Read the model definition and answer for the solid it produces. Units are mm, in the model's axes. Face numbers are marked on the shaded views. A direction names the side the tool comes from. Give positions to 0.01 mm unless a question says otherwise; leave off trailing zeros. Order: outer loops, then holes, each group sorted by start corner. A loop starts at its lowest first (then second) coordinate and runs counter-clockwise, first axis right, second up.
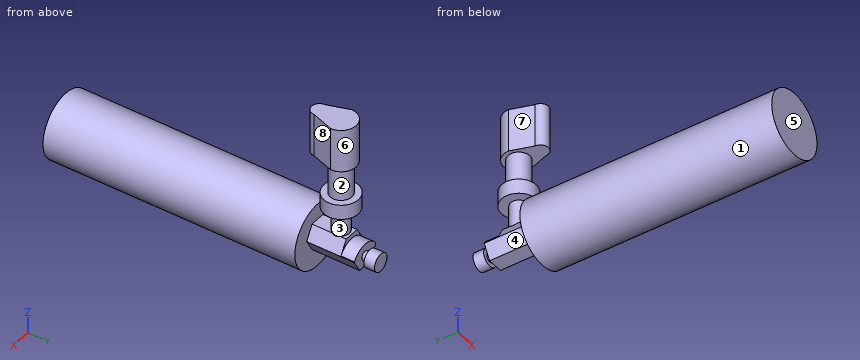
```python
from build123d import *

# Parameters (mm, degrees)
SKETCH1_R                = 14.5
BOSS_EXTRUDE1_DEPTH      = 113.4
SKETCH2_R                = 2
BOSS_EXTRUDE2_DEPTH      = 28.5
SKETCH3_R                = 4
BOSS_EXTRUDE3_DEPTH      = 4.8
BOSS_EXTRUDE4_DEPTH      = 21.4
CUT_EXTRUDE1_DEPTH       = 6
BOSS_EXTRUDE5_DEPTH      = 11
BOSS_EXTRUDE5_DEPTH_BACK = 2
SKETCH7_R                = 3.75
SKETCH8_R                = 7.75
BOSS_EXTRUDE6_DEPTH      = 6.7
SKETCH9_R                = 4.9
BOSS_EXTRUDE7_DEPTH      = 15
BOSS_EXTRUDE8_DEPTH      = 19.5


with BuildPart() as part:
    # Sketch1 → Boss-Extrude1 (new body)
    with BuildSketch(Plane(origin=(0, 0, 0), x_dir=(1, 0, 0), z_dir=(0, 1, 0))):
        with Locations(Location((0, 0, 0), (0, 0, 90))):
            Circle(SKETCH1_R)
    extrude(amount=BOSS_EXTRUDE1_DEPTH)

    # Sketch2 → Boss-Extrude2 (add)
    with BuildSketch(Plane(origin=(0, 113.4, 0), x_dir=(1, 0, 0), z_dir=(0, 1, 0))):
        with Locations(Location((0, 0, 0), (0, 0, 90))):
            Circle(SKETCH2_R)
    extrude(amount=BOSS_EXTRUDE2_DEPTH)

    # Sketch3 → Boss-Extrude3 (add)
    with BuildSketch(Plane(origin=(0, 141.9, 0), x_dir=(1, 0, 0), z_dir=(0, 1, 0))):
        with Locations(Location((0, 0, 0), (0, 0, 270))):
            Circle(SKETCH3_R)
    extrude(amount=-BOSS_EXTRUDE3_DEPTH)

    # Sketch4 → Boss-Extrude4 (add)
    with BuildSketch(Plane(origin=(0, 113.4, 0), x_dir=(1, 0, 0), z_dir=(0, 1, 0))):
        Polygon((3.464101615, 4.7), (-3.464101615, 4.7), (-6.92820323, -1.3), (-3.464101615, -7.3), (3.464101615, -7.3), (6.92820323, -1.3), align=None)
    extrude(amount=BOSS_EXTRUDE4_DEPTH)

    # Sketch6 → Cut-Extrude1 (cut)
    with BuildSketch(Plane(origin=(0, 134.8, 0), x_dir=(1, 0, 0), z_dir=(0, 1, 0))):
        with BuildLine():
            Line((-6.92820323, -1.3), (-6.92820323, -9.46576474))
            Line((-6.92820323, -9.46576474), (6.92820323, -9.46576474))
            Line((6.92820323, -9.46576474), (6.92820323, -1.3))
            ThreePointArc((6.92820323, -1.3), (0, -5.37), (-6.92820323, -1.3))
        make_face()
    extrude(amount=-CUT_EXTRUDE1_DEPTH, mode=Mode.SUBTRACT)

    # Sketch7 → Boss-Extrude5 (add, two sides: drawn at the far end of the back side and taken through both)
    with BuildSketch(Plane.XY.offset(7.3).offset(-BOSS_EXTRUDE5_DEPTH_BACK)):
        with Locations((0, 124.05)):
            Circle(SKETCH7_R)
    extrude(amount=BOSS_EXTRUDE5_DEPTH + BOSS_EXTRUDE5_DEPTH_BACK)

    # Sketch8 → Boss-Extrude6 (add)
    with BuildSketch(Plane.XY.offset(18.3)):
        with Locations((0, 124.05)):
            Circle(SKETCH8_R)
    extrude(amount=BOSS_EXTRUDE6_DEPTH)

    # Sketch9 → Boss-Extrude7 (add)
    with BuildSketch(Plane.XY.offset(25)):
        with Locations((0, 124.05)):
            Circle(SKETCH9_R)
    extrude(amount=BOSS_EXTRUDE7_DEPTH)

    # Sketch10 → Boss-Extrude8 (add)
    with BuildSketch(Plane.XY.offset(40)):
        with BuildLine():
            Line((-6.75, 124.05), (-3.5, 114.3))
            ThreePointArc((-3.5, 114.3), (0, 110.8), (3.5, 114.3))
            Line((3.5, 114.3), (6.75, 124.05))
            ThreePointArc((6.75, 124.05), (0, 130.8), (-6.75, 124.05))
        make_face()
    extrude(amount=BOSS_EXTRUDE8_DEPTH)


solid = part.part
```
1) The part is cut by section B-B on z = 11. Determine the outline of the cut face in (x, y).
Final values:
outline: (-9.45, 0) - (9.45, 0) - (9.45, 113.4) - (-9.45, 113.4) - close; circle Ø7.5 at (0, 124.05)
2) Consider L1, parallel to Y at x = -5, z = -9; L2, parallel to X at y = 105, z = 0; L3, parallel to Z at x = 3.5, y = 84.5. Determine where each line is inside the solid, lowest interval first.
Final values:
L1: y = 0 to 113.4
L2: x = -14.5 to 14.5
L3: z = -14.07 to 14.07
3) A tool of negligible diameter and unlimited length cuts with its end or side. For the marked faces 4, 5, 6, 7 and 8, from which of +Z, -Z, +X, -X, +Y, -Y can it reach the whole face along a straight path? Write none if from no direction.
Final values:
face 4: -Z, -X, +Y
face 5: +Z, -Z, +X, -X, -Y
face 6: +Z, +Y
face 7: +Z, -X, -Y
face 8: +Z, +X, -Y
4) The part is cut by section D-D on z = 46. Determine the outline of the cut face in (x, y), and give its area (3 significant figures).
Final values:
outline: (-6.75, 124.05) - (-3.5, 114.3) arc R3.5 ccw to (3.5, 114.3) - (6.75, 124.05) arc R6.75 ccw to start
area: 191 mm2
5) Given pin 1 (5 mm diameter, centred on y = 103.5, z = 5.5, fed in from -X); pin 2 (8 mm diameter, centred on x = 6, z = 22.5, fed in from +Y); pin 3 (2 mm diameter, centred on x = -5.5, y = 17, fed in from +Z), each flat-ended and moving along its own axis, determine where each tip first touches the part or whether it passes through.
Final values:
pin 1: stops at x = -14.19
pin 2: stops at y = 131.54
pin 3: stops at z = 13.78
6) For a pull along Y with two mould halves and no side action, classify the marked faces 1, 2 and 3 as released by +Y, released by -Y, zero draft, split by the parting line, or undercut.
Final values:
face 1: zero draft
face 2: split by the parting line
face 3: undercut
7) The part is cut by section C-C on y = 74.5. Determine the outline of the cut face in (x, z).
Final values:
outline: circle Ø29 at (0, 0)
